The model under review builds one solid part; all positions refer to its coordinate system, in mm. Face numbers are marked on the shaded views. A direction names the side the tool comes from. Give positions to 0.01 mm unless a question says otherwise; leave off trailing zeros. Order: outer loops, then holes, each group sorted by start corner. A loop starts at its lowest first (then second) coordinate and runs counter-clockwise, first axis right, second up. Notation, with made-up numbers: (24.25, 29) - (30.25, 29) arc R15 cw to (30.25, 52) - close; hole circle Ø1 at (45, 9). An arc over 180 degrees is marked (long way). Put each result on its own line as item: value.
```python
from build123d import *

# Parameters (mm, degrees)
F1_DEPTH = 63.5
F0_W     = 28.575
F0_H     = 19.05
F2_DEPTH = 25.4
F3_DEPTH = 7.9375
F5_R     = 6.35


with BuildPart() as f1:
    # F0 (on Front) → F1 (new body, symmetric)
    with BuildSketch(Plane.XZ):
        Polygon((41.275, -9.525), (41.275, 9.525), (22.225, 9.525), (-41.275, 9.525), (-41.275, -9.525), align=None)
    extrude(amount=F1_DEPTH, both=True)

    # F0 (on Front) → F2 (join, symmetric)
    with BuildSketch(Plane.XZ):
        with BuildLine():
            Line((22.225, 9.525), (41.275, 9.525))
            Line((41.275, 9.525), (41.275, 27.0002))
            ThreePointArc((41.275, 27.0002), (45.9246798487, 38.2255201513), (57.15, 42.8752))
            Line((57.15, 42.8752), (57.15, 61.9252))
            add(Edge.make_bspline(
                [(50.521689096, 61.29044817), (52.7261125358, 61.5243781465), (54.9369393602, 61.735707874), (57.15, 61.9252)],
                knots=[106.439422351, 106.439422351, 106.439422351, 106.439422351, 111.5045361635, 111.5045361635, 111.5045361635, 111.5045361635], degree=3))
            ThreePointArc((50.521689096, 61.29044817), (30.2125782291, 49.2292560605), (22.225, 27.0002))
            Line((22.225, 27.0002), (22.225, 9.525))
        make_face()
        with Locations((71.4375, 52.4002)):
            Rectangle(F0_W, F0_H)
    extrude(amount=F2_DEPTH, both=True)

    # F0 (on Front) → F3 (join, symmetric)
    with BuildSketch(Plane.XZ):
        with BuildLine():
            ThreePointArc((57.15, 61.9252), (53.8206826779, 61.7661498816), (50.521689096, 61.29044817))
            add(Edge.make_bspline(
                [(50.521689096, 61.29044817), (52.7261125358, 61.5243781465), (54.9369393602, 61.735707874), (57.15, 61.9252)],
                knots=[106.439422351, 106.439422351, 106.439422351, 106.439422351, 111.5045361635, 111.5045361635, 111.5045361635, 111.5045361635], degree=3))
        make_face()
        Polygon((41.275, -9.525), (41.275, 9.525), (22.225, 9.525), (-41.275, 9.525), (-41.275, -9.525), align=None)
        with BuildLine():
            Line((-41.275, 9.525), (22.225, 9.525))
            Line((22.225, 9.525), (22.225, 27.0002))
            ThreePointArc((22.225, 27.0002), (30.2125782291, 49.2292560605), (50.521689096, 61.29044817))
            add(Edge.make_bspline(
                [(-41.275, 9.525), (-39.2990761683, 41.4785222008), (4.1974471864, 56.3745918841), (50.521689096, 61.29044817)],
                knots=[0, 0, 0, 0, 106.439422351, 106.439422351, 106.439422351, 106.439422351], degree=3))
        make_face()
    extrude(amount=F3_DEPTH, both=True)

    # F0 (on Front) → F4 (revolve)
    with BuildSketch(Plane.XZ):
        Polygon((85.725, 61.9252), (85.725, 42.8752), (85.725, 38.1), (107.95, 38.1), (107.95, 66.675), (85.725, 66.675), align=None)
    revolve(axis=Axis((85.725, 0, 52.3875), (0, 0, 1)))

    # F5
    f5_edges = [f1.edges().sort_by_distance(p)[0] for p in [
        (-41.275, 63.5, 0),
        (41.275, 63.5, 0),
        (-41.275, -63.5, 0),
        (41.275, -63.5, 0),
    ]]
    fillet(f5_edges, radius=F5_R)


solid = f1.part
```
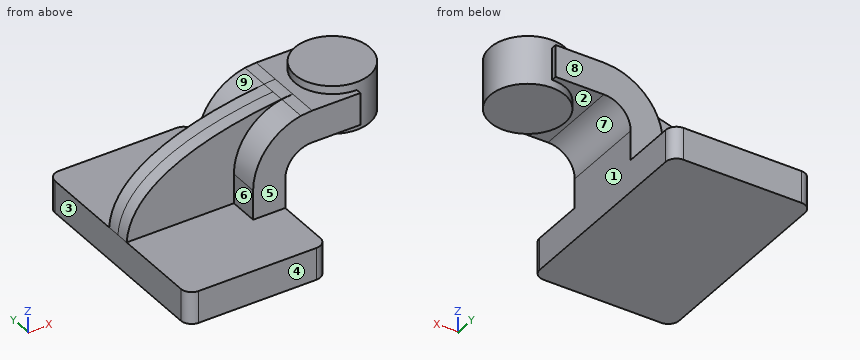
(1) For the marked faces 5, 6, 7, 8 and 9, list the 3-axis set-ups (+Z, -Z, +X, -X, +Y, -Y) from which the entire face can be reached by the end or side of a thin tool; tool diameter is ignored.
The answers:
face 5: +Z, +X, -X, -Y
face 6: +Z, -X, -Y
face 7: -Z, +Y, -Y
face 8: +Z, +X, -X, +Y
face 9: +Z, -X, +Y
(2) Take a section at A-A, the plane z = 7. Write out the cut boundary in (x, y) (3 decimals), then the cut area to 3 significant figures.
The answers:
outline: (-41.275, -57.15) arc R6.35 ccw to (-34.925, -63.5) - (34.925, -63.5) arc R6.35 ccw to (41.275, -57.15) - (41.275, 57.15) arc R6.35 ccw to (34.925, 63.5) - (-34.925, 63.5) arc R6.35 ccw to (-41.275, 57.15) - close
area: 10,400 mm^2
(3) Clearance check with flat-ended pins moving along their axes: pin 1 Ø23 at (x, y) = (72, -7) entering from -Z; pin 2 Ø15.5 at (x, z) = (-14.5, 38.5) entering from +Y; pin 3 Ø18.5 at (y, z) = (-22.5, 14) entering from +X (3 decimals). State where each tip first meets the part, or that it passes through.
The answers:
pin 1: z = 38.1
pin 2: y = 7.94
pin 3: x = 41.275
(4) Wall thickness on L1, parallel to Z at x = 3, y = -49.5 (3 decimals); L2, parallel to Y at x = 14, z = 40; L3, parallel to Z at x = 76, y = 15 (3 decimals): over which ranges is each line inside the solid? List them lowest first.
The answers:
L1: -9.525 to 9.525
L2: -7.94 to 7.94
L3: 38.1 to 66.675
(5) The part is to be moulded in two halves that separate along X. For the marked faces 1, 2, 3 and 4, say which applies: pulls with the +X half, pulls with the -X half, needs draft (parallel to the pull), parting line crosses it, or undercut.
The answers:
face 1: pulls with the +X half
face 2: undercut
face 3: pulls with the -X half
face 4: needs draft
(6) Take a section at B-B, the plane y = -34.5. Write out the cut boundary in (x, z) (3 decimals), then the cut area to 3 significant figures.
The answers:
outline: (-41.275, -9.525) - (41.275, -9.525) - (41.275, 9.525) - (-41.275, 9.525) - close
area: 1,570 mm^2
